Part print with two shaded views. Sizes in mm from the minimum x, y, z corner. A direction names the side the tool comes from. Give positions to 0.01 mm unless a question says otherwise; leave off trailing zeros. Order: outer loops, then holes, each group sorted by start corner. A loop starts at its lowest first (then second) coordinate and runs counter-clockwise, first axis right, second up. Notation, with made-up numbers: M 67,37 L 83,37 A23 ccw 83,46 Z; hole C 62,82 d11. An arc over 180 degrees is marked long. Answer as CSV lines item,"result".
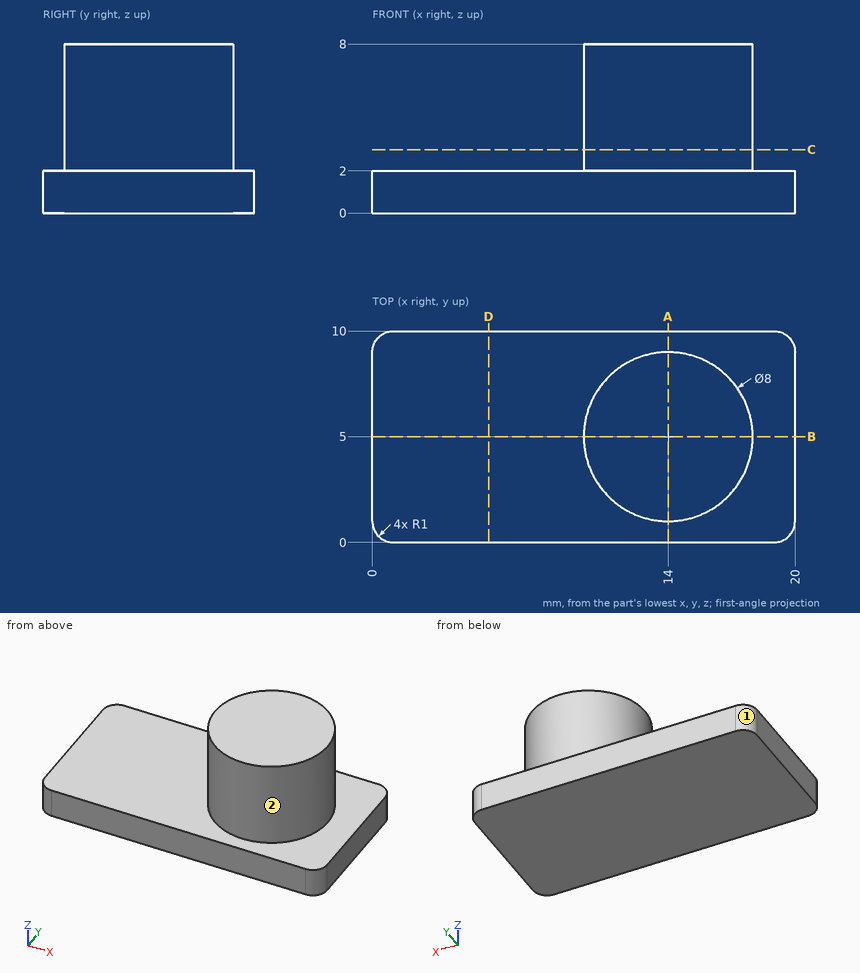
Item 1: Probe line 1 along Z through (x, y) = (3.5, 5.75); line 2 along X through (y, z) = (3.5, 6.5); line 3 along X through (y, z) = (2.25, 2.5). List the from-to ranges inside material, lowest first. Write a range as from..to.
Geometry says:
line 1,"z = 0..2"
line 2,"x = 10.29..17.71"
line 3,"x = 11.1..16.9"
Item 2: Band-saw the part on A-A (x = 14). Give the cut face in (y, z).
Geometry says:
outline,"M 0,0 L 10,0 L 10,2 L 9,2 L 9,8 L 1,8 L 1,2 L 0,2 Z"
Item 3: Band-saw the part on C-C (z = 3). Give the cut face in (x, y).
Geometry says:
outline,"C 14,5 d8"
Item 4: Band-saw the part on D-D (x = 5.5). Give the cut face in (y, z).
Geometry says:
outline,"M 0,0 L 10,0 L 10,2 L 0,2 Z"
Item 5: 3-axis set-ups, long thin cutter, end or side, ignore diameter. For the marked faces 1 and 2: which of +Z, -Z, +X, -X, +Y, -Y reach the whole face in a straight line?
Geometry says:
face 1,"+Z, -Z, -X, +Y"
face 2,"+Z"
Item 6: Band-saw the part on B-B (y = 5). Give the cut face in (x, z), and give its area (3 significant figures).
Geometry says:
outline,"M 0,0 L 20,0 L 20,2 L 18,2 L 18,8 L 10,8 L 10,2 L 0,2 Z"
area,"88.0 mm2"
